Here's how the part is built. I have some questions about the finished solid (model axes, mm). A direction names the side the tool comes from. Coordinates: 2 decimals unless noted, no trailing zeros. Order: outer loops, then holes, each group sorted by start corner. A loop starts at its lowest first (then second) coordinate and runs counter-clockwise, first axis right, second up.
```python
from build123d import *

# Parameters (mm, degrees)
SKETCH_1_R          = 4
EXTRUDE_1_DEPTH     = 6.5
SKETCH_2_W          = 40
SKETCH_2_H          = 3
CUT_EXTRUDE_1_DEPTH = 101.335686573
SKETCH_3_W          = 1
SKETCH_3_H          = 6.5
EXTRUDE_2_DEPTH     = 10


with BuildPart() as part:
    # 草图1 → 凸台-拉伸1 (new body)
    with BuildSketch(Plane(origin=(0, 0, 0), x_dir=(1, 0, 0), z_dir=(0, 1, 0))):
        with BuildLine():
            ThreePointArc((0, 5), (-5, 0), (0, -5))
            Line((0, -5), (40, -5))
            Line((40, -5), (100, -2.5))
            Line((100, -2.5), (100, 2.5))
            Line((100, 2.5), (40, 5))
            Line((40, 5), (0, 5))
        make_face()
        with Locations(Location((0, 0, 0), (0, 0, 90))):
            Circle(SKETCH_1_R, mode=Mode.SUBTRACT)
        with Locations(Location((40, 0, 0), (0, 0, 90))):
            Circle(SKETCH_1_R, mode=Mode.SUBTRACT)
    extrude(amount=EXTRUDE_1_DEPTH)

    # 草图2 → 切除-拉伸1 (cut, through all)
    with BuildSketch(Plane(origin=(0, 6.5, 0), x_dir=(1, 0, 0), z_dir=(0, 1, 0))):
        with Locations((80, 0)):
            Rectangle(SKETCH_2_W, SKETCH_2_H)
    extrude(amount=-CUT_EXTRUDE_1_DEPTH, mode=Mode.SUBTRACT)

    # 草图3 → 凸台-拉伸2 (add)
    with BuildSketch(Plane(origin=(100, 0, 0), x_dir=(0, 0, -1), z_dir=(1, 0, 0))):
        with Locations((-2, 3.25)):
            Rectangle(SKETCH_3_W, SKETCH_3_H)
        with Locations((2, 3.25)):
            Rectangle(SKETCH_3_W, SKETCH_3_H)
    extrude(amount=EXTRUDE_2_DEPTH)


solid = part.part
```
Q1. If we section it at A-A on z = 0: Write out the boundary of the cut face in (x, y).
Q2. For faces 4 (the flat face through (85, 3, 1.5)), 5 (the flat face through (105, 3, 2.5)), 6 (the flat face through (20, 3, -5)), 7 (the flat face through (20, 3, 5)), 8 (the flat face through (105, 3, -2.5)), which set-ups out of +Z, -Z, +X, -X, +Y, -Y let a thin tool reach every point of the face, with its end or its side?
Q3. I need wall thicknesses on L1, parallel to X at y = 3, z = 0; L2, parallel to X at y = 3.25, z = -1.25; L3, parallel to Z at x = 85.5, y = 4.5. Which ranges of each line are inside material? Lowest first, please.
Q4. Will these pins go through, and if not, where does the flat tip stop? pin 1 (0.9 mm diameter, centred on y = 2, z = -0.5, fed in from +X); pin 2 (6 mm diameter, centred on x = 39, z = 2.5, fed in from +Y); pin 3 (2 mm diameter, centred on x = 92, y = 1, fed in from -Z) (3 decimals).
Q5. If we section it at D-D on x = 80: Write out the boundary of the cut face in (y, z), then the cut area to 3 significant figures.
Q6. If we section it at C-C on y = 3.25: Write out the boundary of the cut face in (x, z), then the cut area to 3 significant figures.
Q7. We'd pull the mould along X, two halves only. Please class faces 1 (the cylindrical face through (-5, 3, 0)), 2 (the flat face through (85, 3, -1.5)), 3 (the cylindrical face through (3.905, 3.204, 0.867)): pulls with the +X half, pulls with the -X half, needs draft (parallel to the pull), parting line crosses it, or undercut.
Q8. If we section it at B-B on x = 68: Write out the boundary of the cut face in (y, z), then the cut area to 3 significant figures.
Reply:
1. outline: (-5, 0) - (-4, 0) - (-4, 6.5) - (-5, 6.5) - close; (4, 0) - (36, 0) - (36, 6.5) - (4, 6.5) - close; (44, 0) - (60, 0) - (60, 6.5) - (44, 6.5) - close
2. face 4: +X, +Y, -Y
2. face 5: +Z, +X, +Y, -Y
2. face 6: -Z, +X, -X, +Y, -Y
2. face 7: +Z, +X, -X, +Y, -Y
2. face 8: -Z, +X, +Y, -Y
3. L1: x = -5 to -4, 4 to 36, 44 to 60
3. L2: x = -4.84 to -3.8, 3.8 to 36.2, 43.8 to 60
3. L3: z = -3.1 to -1.5, 1.5 to 3.1
4. pin 1: stops at x = 60
4. pin 2: stops at y = 6.5
4. pin 3: stops at z = -2.875
5. outline: (0, -3.33) - (6.5, -3.33) - (6.5, -1.5) - (0, -1.5) - close; (0, 1.5) - (6.5, 1.5) - (6.5, 3.33) - (0, 3.33) - close
5. area: 23.8 mm2
6. outline: (0, -5) - (40, -5) - (100, -2.5) - (110, -2.5) - (110, -1.5) - (60, -1.5) - (60, 1.5) - (110, 1.5) - (110, 2.5) - (100, 2.5) - (40, 5) - (0, 5) arc R5 ccw to start; hole circle Ø8 at (0, 0); hole circle Ø8 at (40, 0)
6. area: 689 mm2
7. face 1: pulls with the -X half
7. face 2: needs draft
7. face 3: undercut
8. outline: (0, -3.83) - (6.5, -3.83) - (6.5, -1.5) - (0, -1.5) - close; (0, 1.5) - (6.5, 1.5) - (6.5, 3.83) - (0, 3.83) - close
8. area: 30.3 mm2
